CAD build for the part. Positions are in the model's coordinates, mm. Face numbers are marked on the shaded views. A direction names the side the tool comes from. Coordinates: 2 decimals unless noted, no trailing zeros. Loops run counter-clockwise (first coordinate to the right, second up) from the corner with the lowest first, then second, coordinate; pieces in that order, holes last. Notation, with made-up numbers: (79.25, 43.5) -> (136.25, 43.5) arc R23 cw to (136.25, 62.5) -> close; hole circle Ø6 at (86, 56). An arc over 180 degrees is marked (long way). Write each question's results on one line, items separated by ' | '.
```python
from build123d import *

# Parameters (mm, degrees)
MODEL_W             = 5.5
MODEL_H             = 5.5
BOSS_EXTRUDE1_DEPTH = 6


with BuildPart() as part:
    # Model → Boss-Extrude1 (new body)
    with BuildSketch(Plane.XY):
        with BuildLine():
            Line((3357.032259061, 1716.994350869), (3357.032259061, 1710.994350869))
            Line((3357.032259061, 1710.994350869), (3367.032259061, 1710.994350869))
            Line((3367.032259061, 1710.994350869), (3378.032259061, 1710.994350869))
            Line((3378.032259061, 1710.994350869), (3378.032259061, 1741.994350869))
            Line((3378.032259061, 1741.994350869), (3375.536105442, 1741.994350869))
            ThreePointArc((3375.536105442, 1741.994350869), (3408.032259061, 1757.994350869), (3440.528412679, 1741.994350869))
            Line((3440.528412679, 1741.994350869), (3438.032259061, 1741.994350869))
            Line((3438.032259061, 1741.994350869), (3438.032259061, 1710.994350869))
            Line((3438.032259061, 1710.994350869), (3440.532259061, 1710.994350869))
            Line((3440.532259061, 1710.994350869), (3440.532259061, 1704.994350869))
            Line((3440.532259061, 1704.994350869), (3446.532259061, 1704.994350869))
            Line((3446.532259061, 1704.994350869), (3446.532259061, 1710.994350869))
            Line((3446.532259061, 1710.994350869), (3459.032259061, 1710.994350869))
            Line((3459.032259061, 1710.994350869), (3459.032259061, 1716.994350869))
            ThreePointArc((3459.032259061, 1716.994350869), (3408.032259061, 1767.994350869), (3357.032259061, 1716.994350869))
        make_face()
        with Locations((3443.532259061, 1716.494350869)):
            Rectangle(MODEL_W, MODEL_H, mode=Mode.SUBTRACT)
        with Locations((3443.532259061, 1736.494350869)):
            Rectangle(MODEL_W, MODEL_H, mode=Mode.SUBTRACT)
        with Locations((3372.532259061, 1716.494350869)):
            Rectangle(MODEL_W, MODEL_H, mode=Mode.SUBTRACT)
        with Locations((3372.532259061, 1736.494350869)):
            Rectangle(MODEL_W, MODEL_H, mode=Mode.SUBTRACT)
    extrude(amount=BOSS_EXTRUDE1_DEPTH)


solid = part.part
```
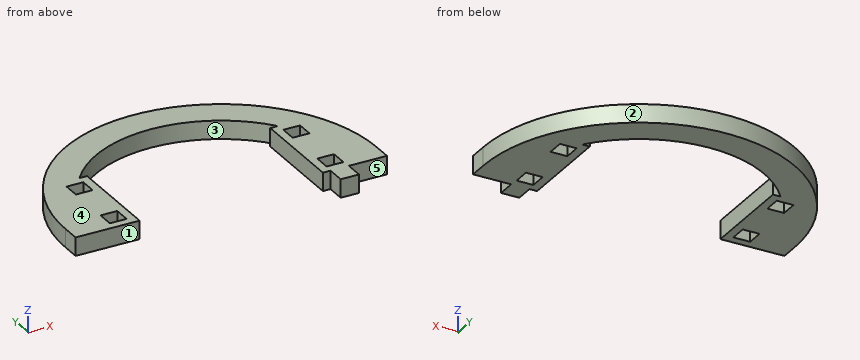
Q1. Cut at B-B on z = 4.9. Give the number of separate pieces and of enclosed holes in the cut face, and give its area (3 significant figures).
Results are:
separate pieces: 1 | enclosed holes: 4 | area: 2,030 mm^2
Q2. Cut at A-A on y = 1731.5. Write the cut outline in (x, z).
Results are:
outline: (3359.14, 0) -> (3378.03, 0) -> (3378.03, 6) -> (3359.14, 6) -> close; (3438.03, 0) -> (3456.93, 0) -> (3456.93, 6) -> (3438.03, 6) -> close
Q3. Cut at C-C on y = 1756.5. Write the cut outline in (x, z).
Results are:
outline: (3375.78, 0) -> (3397.06, 0) -> (3397.06, 6) -> (3375.78, 6) -> close; (3419, 0) -> (3440.29, 0) -> (3440.29, 6) -> (3419, 6) -> close
Q4. Cut at D-D on x = 3425.5. Write the cut outline in (y, z), and give its area (3 significant figures).
Results are:
outline: (1754.09, 0) -> (1764.91, 0) -> (1764.91, 6) -> (1754.09, 6) -> close | area: 64.9 mm^2
Q5. Drop flat-ended pins along their axis: pin 1 (1.8 mm diameter, centred on x = 3454, z = 4, fed in from -Y); pin 2 (3 mm diameter, centred on y = 1737, z = 3, fed in from +X); pin 3 (1.8 mm diameter, centred on y = 1709, z = 3, fed in from +X); pin 4 (4 mm diameter, centred on x = 3387.5, y = 1749.5, fed in from -Z). Give the stop position or say it passes through.
Results are:
pin 1: y = 1710.99 | pin 2: x = 3455.56 | pin 3: x = 3446.53 | pin 4: through
Q6. Which spindle directions (+Z, -Z, +X, -X, +Y, -Y) get a long thin tool onto all of the face, cutting with end or side? Do the marked faces 4 and 5. Say none if no direction does.
Results are:
face 4: +Z, +X, -X, +Y, -Y | face 5: +Z, -Z, +X, -Y
Q7. Pull direction X, two halves, no side cores. Call the marked faces 1, 2 and 3: +X half, -X half, draft (parallel to the pull), parting line (faces both ways), or undercut.
Results are:
face 1: draft | face 2: parting line | face 3: undercut
Q8. Wall check: L1, parallel to X at y = 1716.5, z = 4.7; L2, parallel to X at y = 1739, z = 0.6; L3, parallel to Y at x = 3445.5, z = 5.15. Give the ranges that are in metal, low to high. Write a range as from..to.
Results are:
L1: 3357.03..3369.78, 3375.28..3378.03, 3438.03..3440.78, 3446.28..3459.03 | L2: 3362.02..3369.78, 3375.28..3378.03, 3438.03..3440.78, 3446.28..3454.04 | L3: 1704.99..1713.74, 1719.24..1733.74, 1739.24..1751.59
